Check sheet for the drawn part. Datum: minimum x, y, z corner. Units: mm. A direction names the side the tool comes from. Round coordinates to 2 decimals unless told otherwise and drop trailing zeros. Order: outer loops, then holes, each group sorted by start corner. A loop starts at its lowest first (then second) coordinate and runs counter-clockwise, first axis right, second up. Notation, with made-up numbers: M -24,-34 L 20,-34 A21 cw 20,-13 Z; hole C 64,-20.5 d7. An arc over 180 degrees is marked long. Answer as a JSON object with one key per item and string values. Group by question number.
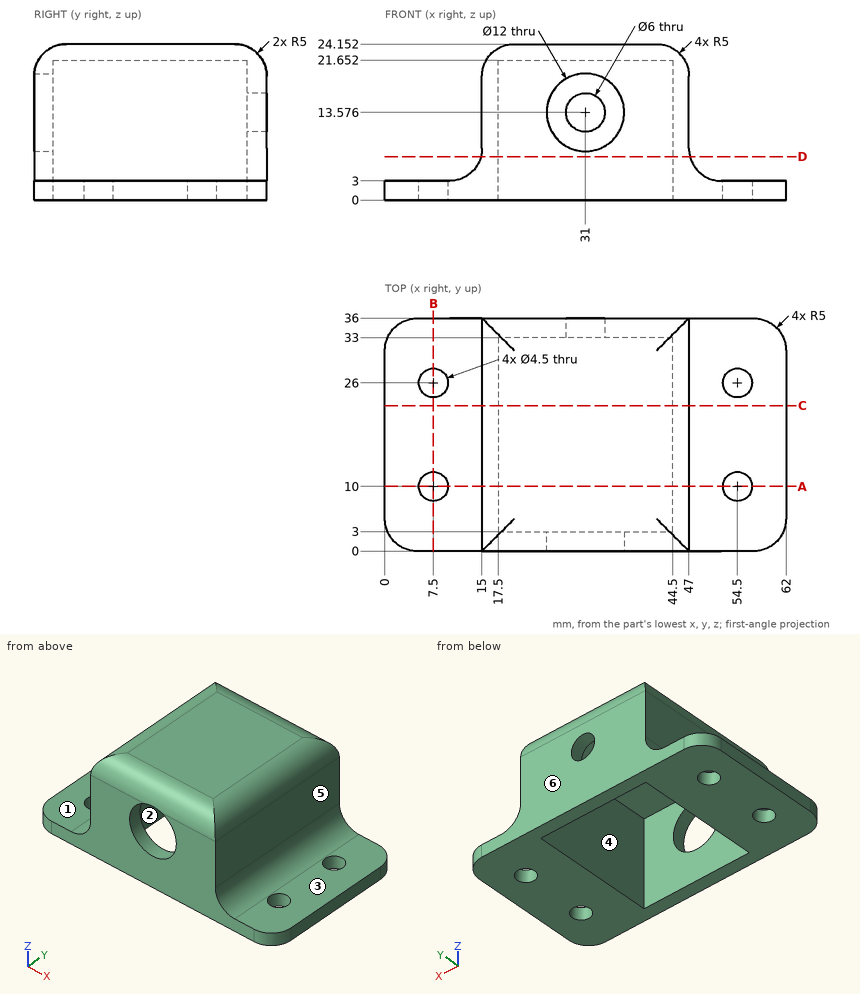
1) Sectioned sample at A-A (y = 10). Record the boundary of the cut face in (x, z).
2) Release check for a two-part mould opening along Y. For the marked faces 4, 5 and 6 record: +Y half, -Y half, draft (parallel to the pull), parting line (faces both ways), or undercut.
3) Go/stop test with flat-tipped pins: P1, Ø10, axis at y = 12, z = 7, coming from the -X side; P2, Ø12, axis at y = 10.5, z = 18.5, coming from the -X side; P3, Ø11, axis at x = 7, y = 23, coming from the +Z side; P4, Ø12.5, axis at y = 11, z = 13, coming from the +X side. Record where each tip stops, or that it passes through.
4) Sectioned sample at D-D (z = 6.75). Record the boundary of the cut face in (x, y), then the cut area to 3 significant figures.
5) Sectioned sample at B-B (x = 7.5). Record the boundary of the cut face in (y, z).
6) Set-up check for the marked faces 1, 2 and 3: record each of +Z, -Z, +X, -X, +Y, -Y from which the full face is reachable in a straight line by a thin tool's end or side.
7) Thickness scan on line 1 along Y through (x, z) = (28, 1.5); line 2 along Y through (x, z) = (54.5, 1.75); line 3 along X through (y, z) = (21.5, 15.5). Record the ranges inside material, lowest first. Write a range as [from, to].
8) Sectioned sample at C-C (y = 22.5). Record the boundary of the cut face in (x, z).
Final values:
{
 "1": {"outline": "M 0,0 L 5.25,0 L 5.25,3 L 0,3 Z; M 9.75,0 L 17.5,0 L 17.5,21.65 L 44.5,21.65 L 44.5,0 L 52.25,0 L 52.25,3 L 52,3 A5 cw 47,8 L 47,19.15 A5 ccw 42,24.15 L 20,24.15 A5 ccw 15,19.15 L 15,8 A5 cw 10,3 L 9.75,3 Z; M 56.75,0 L 62,0 L 62,3 L 56.75,3 Z"},
 "2": {"face 4": "undercut", "face 5": "draft", "face 6": "+Y half"},
 "3": {"P1": "stops at x = 0", "P2": "stops at x = 15", "P3": "stops at z = 3.67", "P4": "stops at x = 47.16"},
 "4": {"outline": "M 14.84,0 L 47.16,0 L 47.16,36 L 14.84,36 Z; hole M 17.5,3 L 44.5,3 L 44.5,33 L 17.5,33 Z", "area": "353 mm^2"},
 "5": {"outline": "M 0,0 L 7.75,0 L 7.75,3 L 0,3 Z; M 12.25,0 L 23.75,0 L 23.75,3 L 12.25,3 Z; M 28.25,0 L 36,0 L 36,3 L 28.25,3 Z"},
 "6": {"face 1": "+Z, -X, +Y, -Y", "face 2": "-Z", "face 3": "+Z, +X, +Y, -Y"},
 "7": {"line 1": "y = [0, 3], [33, 36]", "line 2": "y = [0, 7.75], [12.25, 23.75], [28.25, 36]", "line 3": "x = [15, 17.5], [44.5, 47]"},
 "8": {"outline": "M 0,0 L 17.5,0 L 17.5,21.65 L 44.5,21.65 L 44.5,0 L 62,0 L 62,3 L 52,3 A5 cw 47,8 L 47,19.15 A5 ccw 42,24.15 L 20,24.15 A5 ccw 15,19.15 L 15,8 A5 cw 10,3 L 0,3 Z"}
}
